from build123d import *

# Parameters (mm, degrees)
BOSS_EXTRUDE2_DEPTH = 1.7
BOSS_EXTRUDE3_DEPTH = 3


with BuildPart() as part:
    # Sketch3 → Boss-Extrude2 (new body)
    with BuildSketch(Plane(origin=(0, 0, 0), x_dir=(1, 0, 0), z_dir=(0, 1, 0))):
        Polygon((0, -83.094010768), (71.961524227, -41.547005384), (71.961524227, 41.547005384), (0, 83.094010768), (-71.961524227, 41.547005384), (-71.961524227, -41.547005384), align=None)
        Polygon((-1.192537669, 54.404010768), (-46.518986558, 28.2347733), (-47.711524227, 26.169237467), (-47.711524227, -26.169237467), (-46.518986558, -28.2347733), (-1.192537669, -54.404010768), (1.192537669, -54.404010768), (46.518986558, -28.2347733), (47.711524227, -26.169237467), (47.711524227, 26.169237467), (46.518986558, 28.2347733), (1.192537669, 54.404010768), align=None, mode=Mode.SUBTRACT)
    extrude(amount=BOSS_EXTRUDE2_DEPTH)

    # Sketch6 → Boss-Extrude3 (add)
    with BuildSketch(Plane.XZ):
        Polygon((0, 83.094010768), (-71.961524227, 41.547005384), (-71.961524227, -41.547005384), (0, -83.094010768), (71.961524227, -41.547005384), (71.961524227, 41.547005384), align=None)
    extrude(amount=BOSS_EXTRUDE3_DEPTH)


solid = part.part
Model file for the job. Use its own axes, mm. A direction names the side the tool comes from. Round coordinates to 2 decimals unless told otherwise and drop trailing zeros. Order: outer loops, then holes, each group sorted by start corner. A loop starts at its lowest first (then second) coordinate and runs counter-clockwise, first axis right, second up.
(1) Band-saw the part on C-C (x = -35). List the corners of the cut face in (y, z), then the cut area to 3 significant figures.
(2) Pin check, flat tips, straight feed: pin 1 (2 mm diameter, centred on x = 22.5, y = 0, fed in from -Z); pin 2 (0.8 mm diameter, centred on x = 0.5, y = 1, fed in from -Z); pin 3 (1.5 mm diameter, centred on x = 6, y = -1.5, fed in from +Z). Stop position of each tip, or through.
(3) 3-axis set-ups, long thin cutter, end or side, ignore diameter. For faces 1 (the face through (-35.5, -0.6, 62.6)), 2 (the face through (-23.54, 0.84, -41.5)): which of +Z, -Z, +X, -X, +Y, -Y reach the whole face in a straight line?
(4) Band-saw the part on D-D (z = -57). List the corners of the cut face in (x, y).
(5) Drill centre lines: line 1 (Y direction, x = 11.5, z = 43); line 2 (X direction, y = 1.2, z = -25); line 3 (Z direction, x = 45.5, y = 0.25). Where is each one in solid material? Low to high.
(6) Band-saw the part on B-B (z = 8.5). List the corners of the cut face in (x, y).
(7) Band-saw the part on A-A (y = 0.9). List the corners of the cut face in (x, z).
(8) Pull direction Z, two halves, no side cores. Call faces 3 (the face through (23.54, 0.84, 41.5)), 4 (the face through (-71.962, -1, 1)), 5 (the face through (35.5, -0.6, -62.6)), 6 (the face through (-24.17, 0.84, 41.14)): released by +Z, released by -Z, zero draft, split by the parting line, or undercut.
Verdict:
1. outline: (-3, -62.89) - (1.7, -62.89) - (1.7, -34.89) - (0, -34.89) - (0, 34.89) - (1.7, 34.89) - (1.7, 62.89) - (-3, 62.89) - close
1. area: 473 mm2
2. pin 1: stops at z = -70.68
2. pin 2: stops at z = -83.04
2. pin 3: stops at z = 80.06
3. face 1: +Z, -X, +Y, -Y
3. face 2: +Y
4. outline: (-45.2, -3) - (45.2, -3) - (45.2, 1.7) - (-45.2, 1.7) - close
5. line 1: y = -3 to 0
5. line 2: x = -71.96 to -47.71, 47.71 to 71.96
5. line 3: z = -56.82 to -28.82, 28.82 to 56.82
6. outline: (-71.96, -3) - (71.96, -3) - (71.96, 1.7) - (47.71, 1.7) - (47.71, 0) - (-47.71, 0) - (-47.71, 1.7) - (-71.96, 1.7) - close
7. outline: (-71.96, -41.55) - (0, -83.09) - (71.96, -41.55) - (71.96, 41.55) - (0, 83.09) - (-71.96, 41.55) - close; hole (-47.71, -26.17) - (-46.52, -28.23) - (-1.19, -54.4) - (1.19, -54.4) - (46.52, -28.23) - (47.71, -26.17) - (47.71, 26.17) - (46.52, 28.23) - (1.19, 54.4) - (-1.19, 54.4) - (-46.52, 28.23) - (-47.71, 26.17) - close
8. face 3: undercut
8. face 4: zero draft
8. face 5: released by -Z
8. face 6: undercut
